Autodesk Inventor part; units mm, degrees
ref_plane "YZ Plane" through (0, 0, 0) normal (1, 0, 0) x (0, 1, 0)
ref_plane "XZ Plane" through (0, 0, 0) normal (0, 1, 0) x (-1, 0, 0)
ref_plane "XY Plane" through (0, 0, 0) normal (0, 0, 1) x (1, 0, 0)
sketch "Sketch1" plane through (0, 0, 0) normal (0, 1, 0) x (-1, 0, 0)
  line L0 (0, 0) -> (0, 150)
  line L1 (0, 150) -> (125, 150)
  line L2 (125, 150) -> (125, -150)
  line L3 (125, -150) -> (-125, -150)
  line L4 (-125, -150) -> (-125, 150)
  line L5 (-125, 150) -> (0, 150)
  line L6 (125, 150) -> (125, 140)
  line L7 (125, 140) -> (115, 140)
  circle A0 centre (115, 140) radius 5
  line L8 (125, 0) -> (-125, 0)
  line L9 (0, 150) -> (0, -150)
  circle A1 centre (115, -140) radius 5
  circle A2 centre (-115, 140) radius 5
  circle A3 centre (-115, -140) radius 5
  dimension "d0" = 150
  dimension "d1" = 125
  dimension "d2" = 300
  dimension "d3" = 250
  dimension "d4" = 10
  dimension "d5" = 10
  dimension "d6" = 10
extrude "Extrusion1" add sketch "Sketch1" along normal blind 10
fillet "Fillet1" radius 5 4 edges at (-125, 5, 150) (-125, 5, -150) (125, 5, -150) (125, 5, 150)
sketch "Sketch2" plane through (0, 10, 0) normal (0, 1, 0) x (1, 0, 0)
  line L0 (-120, -150) -> (120, -150)
  line L1 (-117.475, -150) -> (-117.475, -145)
  line L2 (125, -145) -> (125, 145)
  line L3 (-117.475, -145) -> (125, -145)
  line L4 (0, 0) -> (0, -145)
  line L5 (0, -145) -> (-20, -145)
  line L6 (-20, -145) -> (-20, -125)
  line L7 (-20, -125) -> (20, -125)
  line L8 (20, -125) -> (20, -145)
  line L9 (-125, 145) -> (-125, -145)
  line L10 (-125, 0) -> (125, 0)
  line L11 (-117.475, 145) -> (125, 145)
  line L12 (-20, 145) -> (-20, 125)
  line L13 (-20, 125) -> (20, 125)
  line L14 (20, 125) -> (20, 145)
  dimension "d10" = 5
  dimension "d11" = 20
  dimension "d12" = 20
  dimension "d13" = 40
extrude "Extrusion2" add sketch "Sketch2" along normal blind 30 contours L14 L13 L12 L11 | L3 L4 L7 L8 | L3 L6 L7 L4
fillet "Fillet2" radius 5 10 edges at (-20, 40, -135) (20, 40, -135) (-20, 40, 135) (20, 40, 135) (20, 25, 125) (20, 25, -125) (-20, 25, -125) (-20, 25, 125) (0, 40, 125) (0, 40, -125)
sketch "Sketch3" plane through (20, 10, -145) normal (0, 0, -1) x (-1, 0, 0)
  line L0 (40, 0) -> (40, 25)
  line L1 (40, 0) -> (20, 0)
  line L2 (140, 0) -> (-100, 0)
  line L3 (20, 0) -> (20, 15)
  circle A0 centre (20, 15) radius 3
  point P0 (20, -10)
  dimension "d17" = 20
  dimension "d18" = 15
  dimension "d19" = 6
hole "Hole1" at (0, 25, -145) direction (0, 0, 1) diameter 6 end through all
sketch "Sketch4" plane through (0, 10, 0) normal (0, 1, 0) x (1, 0, 0)
  line L0 (125, -145) -> (125, 145)
  line L1 (125, 0) -> (105, 0)
  line L2 (105, 0) -> (105, -60)
  line L3 (105, -60) -> (55, -60)
  line L4 (55, -60) -> (55, 60)
  line L5 (55, 60) -> (105, 60)
  line L6 (105, 60) -> (105, 0)
  line L7 (105, 0) -> (80, 0)
  line L8 (80, 0) -> (80, -70)
  circle A0 centre (80, -70) radius 2
  circle A1 centre (80, 70) radius 2
  point P0 (0, 0)
  dimension "d27" = 20
  dimension "d28" = 60
  dimension "d29" = 50
  dimension "d30" = 120
  dimension "d31" = 25
  dimension "d32" = 70
  dimension "d33" = 4
extrude "Extrusion3" cut sketch "Sketch4" against normal blind 30
sketch "Sketch5" plane through (0, 0, 0) normal (0, -1, 0) x (1, 0, 0)
  line L0 (-125, -145) -> (-125, 145)
  line L1 (-125, 0) -> (-35, 0)
  line L2 (-35, 0) -> (-35, -120.65)
  line L3 (-35, -120.65) -> (-35, 114.35)
  line L4 (-35, -120.65) -> (-35, -84.15)
  line L5 (-35, -101.6) -> (-65, -101.6)
  line L6 (-65, -101.6) -> (-5, -101.6)
  line L7 (-65, -101.6) -> (-65, -81.6)
  line L8 (-65, -81.6) -> (-5, -81.6)
  line L9 (-5, -81.6) -> (-5, -101.6)
  line L10 (-35, -81.6) -> (-35, -14.85)
  circle A0 centre (-35, -14.85) radius 17.5
  line L11 (-35, 2.6) -> (-35, 118.15)
  circle A1 centre (-35, 118.15) radius 7.5
  point P0 (0, 0)
  dimension "d36" = 90
  dimension "d37" = 235
  dimension "d38" = 36.5
  dimension "d39" = 30
  dimension "d40" = 60
  dimension "d41" = 20
  dimension "d42" = 66.75
  dimension "d43" = 35
  dimension "d44" = 115.55
  dimension "d45" = 15
extrude "Extrusion4" cut sketch "Sketch5" against normal blind 10
properties part number "top"
For this review, take the finished solid that the model builds, in its own axes (mm). A direction names the side the tool comes from. Round coordinates to 2 decimals unless told otherwise and drop trailing zeros. Write each loop counter-clockwise with the first axis right and the second up, starting at its lowest first coordinate (ties: lowest second). Pieces come first, ordered by that corner, then holes.
1) Take a section at C-C on y = 18. Give the boundary of the cut face in (x, z), then the cut area to 3 significant figures.
Answer below:
outline: (-20, -145) - (20, -145) - (20, -130) arc R5 ccw to (15, -125) - (-15, -125) arc R5 ccw to (-20, -130) - close; (-20, 130) arc R5 ccw to (-15, 125) - (15, 125) arc R5 ccw to (20, 130) - (20, 145) - (-20, 145) - close
area: 1,580 mm2
2) Insertion check: pin 1 Ø12 at (x, z) = (-49.5, -97) entering from +Y; pin 2 Ø12.5 at (x, y) = (6.5, 22.5) entering from -Z; pin 3 Ø4.5 at (y, z) = (26, 140.5) entering from -X. Each pin has a flat end and moves straight along its axis. Give the tip position at first contact, or say it passes through.
Answer below:
pin 1: stops at y = 10
pin 2: stops at z = -145
pin 3: stops at x = -20
3) Machinability: for faces 1 (the face through (0, 21, -145)), 2 (the face through (-5, 5, -91)), 3 (the face through (20, 22, -137)), 4 (the face through (0, 20, 125)), which of the approach directions +Z, -Z, +X, -X, +Y, -Y give a long, thin tool a straight path to every point of the face, cutting with its end or side? Answer none if there is none.
Answer below:
face 1: -Z, +X, -X, +Y
face 2: +Y, -Y
face 3: +Z, -Z, +X, +Y
face 4: +X, -X, +Y
4) Mouldability with a two-part tool opening along X and no side actions: class faces 5 (the face through (-20, 22, 138)), 6 (the face through (0, 40, -138)), 7 (the face through (80, 5, -60)) as +X half, -X half, draft (parallel to the pull), parting line (faces both ways), or undercut.
Answer below:
face 5: -X half
face 6: draft
face 7: undercut
5) Take a section at B-B on x = 115. Give the boundary of the cut face in (y, z).
Answer below:
outline: (0, -150) - (10, -150) - (10, -145) - (0, -145) - close; (0, -135) - (10, -135) - (10, 135) - (0, 135) - close; (0, 145) - (10, 145) - (10, 150) - (0, 150) - close
6) For line 1 along Z through (x, y) = (80, 5); line 2 along X through (y, z) = (7, -14); line 3 along Z through (x, y) = (115, 6), list the stretches that pass through material, from the lowest coordinate up.
Answer below:
line 1: z = -150 to -72, -68 to -60, 60 to 68, 72 to 150
line 2: x = -125 to -52.48, -17.52 to 55, 105 to 125
line 3: z = -150 to -145, -135 to 135, 145 to 150
7) Take a section at D-D on z = -43. Give the boundary of the cut face in (x, y), then the cut area to 3 significant figures.
Answer below:
outline: (-125, 0) - (55, 0) - (55, 10) - (-125, 10) - close; (105, 0) - (125, 0) - (125, 10) - (105, 10) - close
area: 2,000 mm2
8) Take a section at A-A on z = 140. Give the boundary of the cut face in (x, y).
Answer below:
outline: (-125, 0) - (-120, 0) - (-120, 10) - (-125, 10) - close; (-110, 0) - (110, 0) - (110, 10) - (20, 10) - (20, 35) arc R5 ccw to (15, 40) - (-15, 40) arc R5 ccw to (-20, 35) - (-20, 10) - (-110, 10) - close; (120, 0) - (125, 0) - (125, 10) - (120, 10) - close; hole circle Ø6 at (0, 25)
